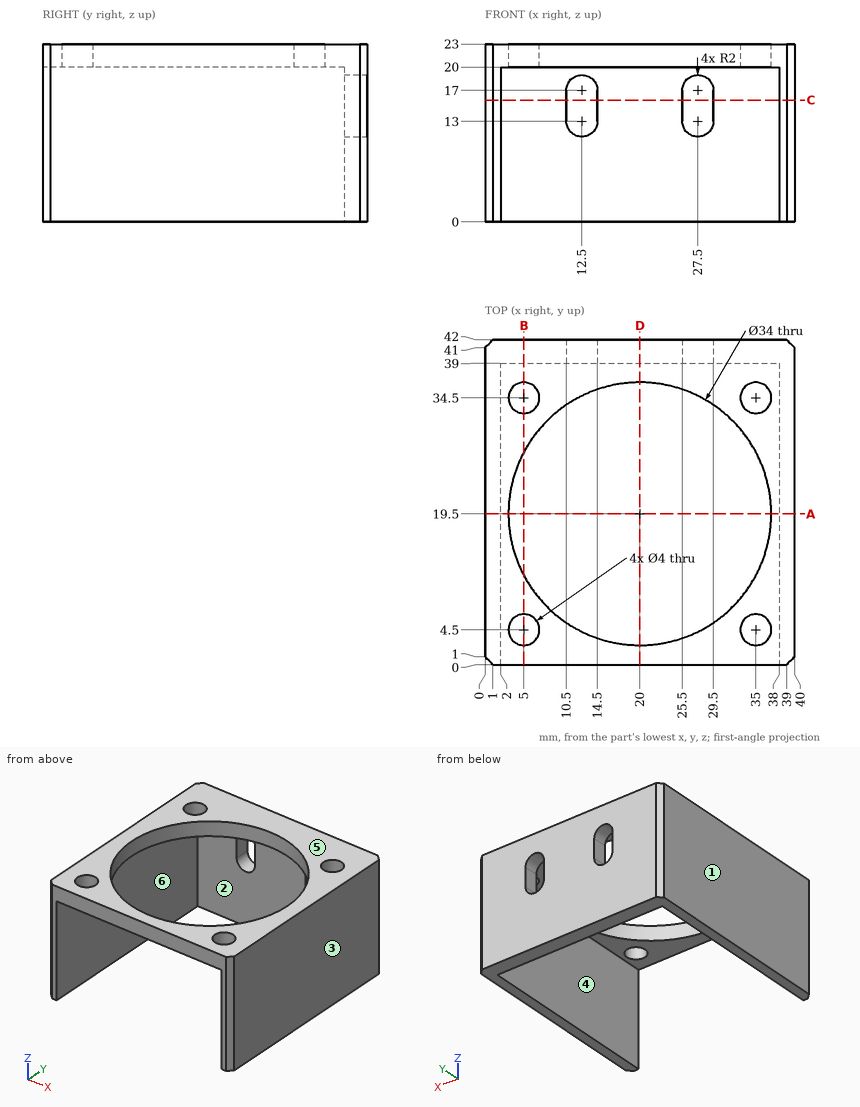
Could you check a few things on this drawing? It's one solid part, dimensions in mm from its lowest x, y, z. A direction names the side the tool comes from. Coordinates: 2 decimals unless noted, no trailing zeros. Order: outer loops, then holes, each group sorted by start corner. A loop starts at its lowest first (then second) coordinate and runs counter-clockwise, first axis right, second up.
1) We'd pull the mould along X, two halves only. Please class the marked faces 1, 2, 3 and 4: +X half, -X half, draft (parallel to the pull), parting line (faces both ways), or undercut.
2) Imagine slicing it at A-A on y = 19.5. List the corners of the cut face in (x, z) for me.
3) Imagine slicing it at B-B on x = 5. List the corners of the cut face in (y, z) for me.
4) I need wall thicknesses on line 1 (X direction, y = 2, z = 19.75); line 2 (Y direction, x = 5, z = 21.8); line 3 (Y direction, x = 20, z = 22). Which ranges of each line are inside material? Lowest first, please.
5) Will these pins go through, and if not, where does the flat tip stop? pin 1 (10 mm diameter, centred on x = 14, z = 10.5, fed in from -Y); pin 2 (8 mm diameter, centred on x = 21.5, y = 32.5, fed in from -Z).
6) Which directions (+Z, -Z, +X, -X, +Y, -Y) give clear straight access to the entire face, cutting with the end or side of a thin tool? Please do the marked faces 5 and 6.
7) Imagine slicing it at D-D on x = 20. List the corners of the cut face in (y, z) for me.
8) Imagine slicing it at C-C on z = 15.75. List the corners of the cut face in (x, y) for me.
Response values:
1. face 1: -X half
1. face 2: undercut
1. face 3: +X half
1. face 4: undercut
2. outline: (0, 0) - (2, 0) - (2, 20) - (3, 20) - (3, 23) - (0, 23) - close; (37, 20) - (38, 20) - (38, 0) - (40, 0) - (40, 23) - (37, 23) - close
3. outline: (0, 20) - (2.5, 20) - (2.5, 23) - (0, 23) - close; (6.5, 20) - (11.5, 20) - (11.5, 23) - (6.5, 23) - close; (27.5, 20) - (32.5, 20) - (32.5, 23) - (27.5, 23) - close; (36.5, 20) - (39, 20) - (39, 0) - (42, 0) - (42, 23) - (36.5, 23) - close
4. line 1: x = 0 to 2, 38 to 40
4. line 2: y = 0 to 2.5, 6.5 to 11.5, 27.5 to 32.5, 36.5 to 42
4. line 3: y = 0 to 2.5, 36.5 to 42
5. pin 1: stops at y = 39
5. pin 2: stops at z = 20
6. face 5: +Z, +X, -X, +Y, -Y
6. face 6: -Z, -Y
7. outline: (0, 20) - (2.5, 20) - (2.5, 23) - (0, 23) - close; (36.5, 20) - (39, 20) - (39, 0) - (42, 0) - (42, 23) - (36.5, 23) - close
8. outline: (0, 1) - (1, 0) - (2, 0) - (2, 39) - (10.5, 39) - (10.5, 42) - (1, 42) - (0, 41) - close; (14.5, 39) - (25.5, 39) - (25.5, 42) - (14.5, 42) - close; (29.5, 39) - (38, 39) - (38, 0) - (39, 0) - (40, 1) - (40, 41) - (39, 42) - (29.5, 42) - close
